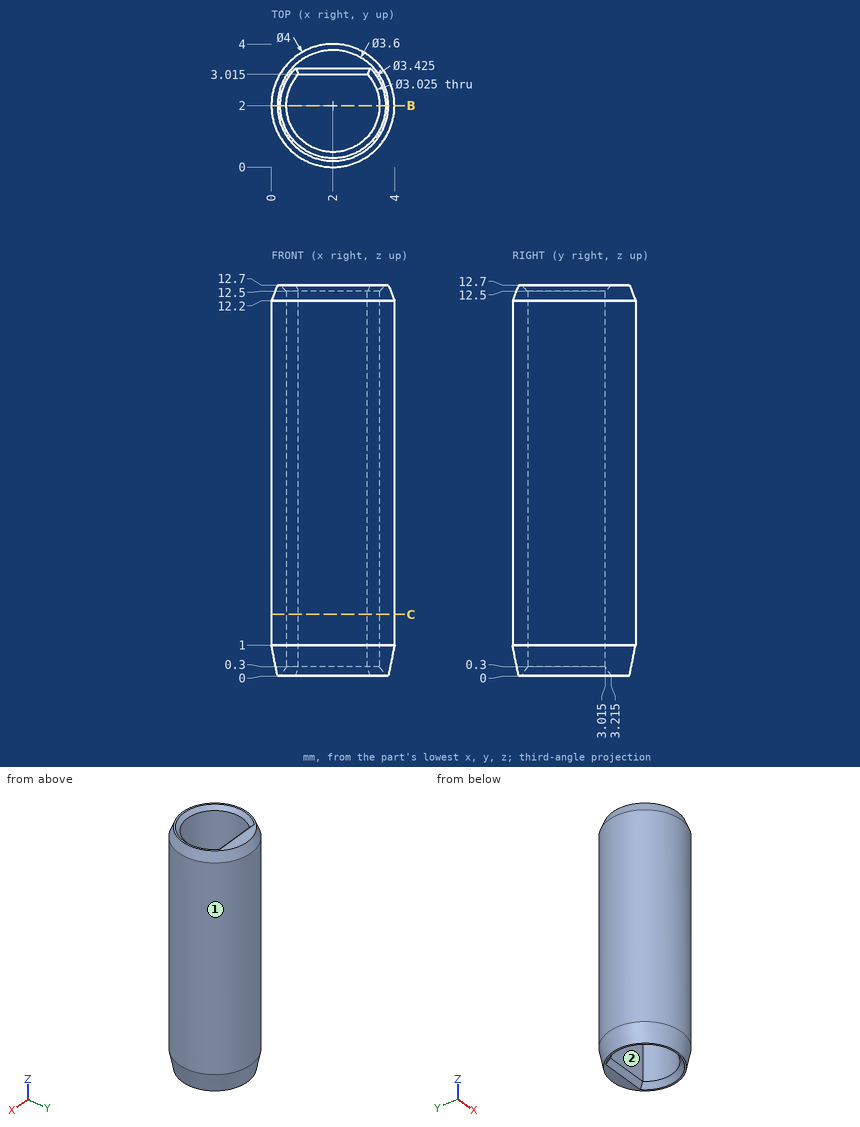
Verification items for this drawing (mm, ordinates from the low corner). Round coordinates to 2 decimals unless told otherwise and drop trailing zeros. Write each loop counter-clockwise with the first axis right and the second up, starting at its lowest first coordinate (ties: lowest second). Pieces come first, ordered by that corner, then holes. Notation, with made-up numbers: (-16.5, 18) - (23.5, 18) arc R23 cw to (23.5, 49) - close; hole circle Ø4 at (88.25, 89.25). An arc over 180 degrees is marked (long way). One line per item, written item: value.
1. Cross-section at B-B on y = 2. Record the boundary of the cut face in (x, z).
The answers:
outline: (0, 1) - (0.2, 0) - (0.29, 0) - (0.49, 0.3) - (0.49, 12.5) - (0.29, 12.7) - (0.2, 12.7) - (0, 12.2) - close; (3.51, 0.3) - (3.71, 0) - (3.8, 0) - (4, 1) - (4, 12.2) - (3.8, 12.7) - (3.71, 12.7) - (3.51, 12.5) - close
2. Scan lines: L1, parallel to Y at x = 2, z = 6 (1 decimal); L2, parallel to X at y = 2.2, z = 7; L3, parallel to Y at x = 2.75, z = 5.25 (3 decimals). Record each from-to range of solid material in increasing order.
The answers:
L1: y = 0 to 0.5, 3 to 4
L2: x = 0.01 to 0.5, 3.5 to 3.99
L3: y = 0.146 to 0.687, 3.015 to 3.854
3. Mould release check, pull along X, two halves, no side actions. Record for the marked faces 1 and 2: released by +X, released by -X, zero draft, split by the parting line, or undercut.
The answers:
face 1: split by the parting line
face 2: undercut
4. Cross-section at C-C on z = 2. Record the boundary of the cut face in (x, y) (1 decimal), and give its area (3 significant figures).
The answers:
outline: circle Ø4 at (2, 2); hole (0.9, 3) arc R1.5 ccw (long way) to (3.1, 3) - close
area: 6.15 mm^2
